from build123d import *

# Parameters (mm, degrees)
ESTRUSIONE_ESTRUSIONE1_DEPTH = 5
ESTRUSIONE_ESTRUSIONE2_DEPTH = 7
ESTRUSIONE_ESTRUSIONE3_DEPTH = 2
ESTRUSIONE_ESTRUSIONE4_DEPTH = 52
TAGLIO_ESTRUSIONE2_DEPTH     = 52
ESTRUSIONE_ESTRUSIONE5_DEPTH = 9
FORI_FILETTATI_3_0MM1_D      = 3


with BuildPart() as part:
    # Schizzo1 → Estrusione-Estrusione1 (new body)
    with BuildSketch(Plane.XY):
        with BuildLine():
            Line((-82.995904107, -166.584374689), (-92.877799089, -168.116742646))
            ThreePointArc((-92.877799089, -168.116742646), (-110.220012955, -164.040092202), (-119.840608042, -149.046239769))
            ThreePointArc((-119.840608042, -149.046239769), (-118.364815633, -130.917411526), (-107.867932944, -116.063192243))
            Line((-107.867932944, -116.063192243), (-84.49215827, -97.259651129))
            ThreePointArc((-84.49215827, -97.259651129), (-67.733683115, -90.189581316), (-49.709718148, -92.632748029))
            ThreePointArc((-49.709718148, -92.632748029), (-37.125664022, -105.242785395), (-36.859828578, -123.055724291))
            Line((-36.859828578, -123.055724291), (-40.474113425, -132.379722631))
            Line((-40.474113425, -132.379722631), (-54.467826156, -126.955304689))
            Line((-54.467826156, -126.955304689), (-50.853541308, -117.631306349))
            ThreePointArc((-50.853541308, -117.631306349), (-51.095893898, -108.22813541), (-57.953355129, -101.789689638))
            ThreePointArc((-57.953355129, -101.789689638), (-68.520842721, -100.735914417), (-78.224311232, -105.051576021))
            Line((-78.224311232, -105.051576021), (-101.600085906, -123.855117134))
            ThreePointArc((-101.600085906, -123.855117134), (-107.894780127, -132.408424149), (-109.129903142, -142.956253658))
            ThreePointArc((-109.129903142, -142.956253658), (-104.310440062, -151.034071069), (-95.177618995, -153.285723315))
            Line((-95.177618995, -153.285723315), (-85.295724012, -151.753355358))
            Line((-85.295724012, -151.753355358), (-82.995904107, -166.584374689))
        make_face()
    extrude(amount=ESTRUSIONE_ESTRUSIONE1_DEPTH)

    # Schizzo2 → Estrusione-Estrusione2 (add)
    with BuildSketch(Plane.XY.offset(5)):
        with BuildLine():
            Line((-36.859828578, -123.055724291), (-50.830842779, -117.640105037))
            ThreePointArc((-50.830842779, -117.640105037), (-50.298673229, -115.886666013), (-50.034997321, -114.073318872))
            Line((-50.034997321, -114.073318872), (-35.811832194, -119.586680021))
            ThreePointArc((-35.811832194, -119.586680021), (-36.269524014, -121.341233275), (-36.859828578, -123.055724291))
        make_face()
        with BuildLine():
            Line((-96.490830562, -168.397042736), (-98.828360202, -153.322841843))
            ThreePointArc((-98.828360202, -153.322841843), (-97.000632762, -153.453858051), (-95.173888567, -153.309779998))
            Line((-95.173888567, -153.309779998), (-92.877799089, -168.116742646))
            ThreePointArc((-92.877799089, -168.116742646), (-94.678957246, -168.325951195), (-96.490830562, -168.397042736))
        make_face()
    extrude(amount=ESTRUSIONE_ESTRUSIONE2_DEPTH)

    # Schizzo3 → Estrusione-Estrusione3 (add)
    with BuildSketch(Plane.XY.offset(12)):
        with BuildLine():
            Line((-42.270578454, -137.014176653), (-36.859828578, -123.055724291))
            ThreePointArc((-36.859828578, -123.055724291), (-36.269524014, -121.341233275), (-35.811832194, -119.586680021))
            Line((-35.811832194, -119.586680021), (-50.034997321, -114.073318872))
            ThreePointArc((-50.034997321, -114.073318872), (-50.288758238, -115.888878313), (-50.830842779, -117.640105037))
            Line((-50.830842779, -117.640105037), (-53.115040991, -123.532795079))
            Line((-53.115040991, -123.532795079), (-42.270578454, -137.014176653))
        make_face()
        with BuildLine():
            Line((-96.490830562, -168.397042736), (-98.828360202, -153.322841843))
            ThreePointArc((-98.828360202, -153.322841843), (-97.000596453, -153.464016791), (-95.173888567, -153.309779998))
            Line((-95.173888567, -153.309779998), (-88.928612449, -152.34133609))
            Line((-88.928612449, -152.34133609), (-78.084149913, -165.822717664))
            Line((-78.084149913, -165.822717664), (-92.877799089, -168.116742646))
            ThreePointArc((-92.877799089, -168.116742646), (-94.678957246, -168.325951195), (-96.490830562, -168.397042736))
        make_face()
    extrude(amount=ESTRUSIONE_ESTRUSIONE3_DEPTH)

    # Schizzo4 → Estrusione-Estrusione4 (add)
    with BuildSketch(Plane.XY.offset(5)):
        Polygon((-101.600085906, -123.855117134), (-78.224311232, -105.051576021), (-84.49215827, -97.259651129), (-107.867932944, -116.063192243), align=None)
    extrude(amount=ESTRUSIONE_ESTRUSIONE4_DEPTH)

    # Schizzo5 → Taglio-Estrusione2 (cut)
    with BuildSketch(Plane.XY.offset(57)):
        Polygon((-97.246900104, -116.503262037), (-97.873684808, -115.724069548), (-98.141552252, -109.009291291), (-98.517623074, -108.541775798), (-93.842468139, -104.781067575), (-93.466397317, -105.248583068), (-86.96498996, -106.949083694), (-86.338205256, -107.728276184), align=None)
    extrude(amount=-TAGLIO_ESTRUSIONE2_DEPTH, mode=Mode.SUBTRACT)

    # Schizzo6 → Estrusione-Estrusione5 (add)
    with BuildSketch(Plane.XY.offset(5)):
        with BuildLine():
            Line((-105.360794128, -119.1799622), (-104.107224721, -120.738347178))
            ThreePointArc((-104.107224721, -120.738347178), (-113.327097811, -135.89060806), (-110.731703589, -153.436576214))
            ThreePointArc((-110.731703589, -153.436576214), (-105.298812913, -158.702833766), (-97.823256998, -159.87152255))
            Line((-97.823256998, -159.87152255), (-97.519846298, -161.848374074))
            ThreePointArc((-97.519846298, -161.848374074), (-106.191101066, -160.49275607), (-112.492970749, -154.384172115))
            ThreePointArc((-112.492970749, -154.384172115), (-115.28727508, -135.493487076), (-105.360794128, -119.1799622))
        make_face()
        with BuildLine():
            Line((-43.853805634, -116.458338954), (-41.987888093, -117.178305432))
            ThreePointArc((-41.987888093, -117.178305432), (-41.453924934, -108.417983362), (-46.070241465, -100.953535552))
            ThreePointArc((-46.070241465, -100.953535552), (-63.923362402, -94.176206375), (-81.985019455, -100.376421086))
            Line((-81.985019455, -100.376421086), (-80.731450047, -101.934806064))
            ThreePointArc((-80.731450047, -101.934806064), (-63.955496248, -96.175948212), (-47.373234104, -102.470839142))
            ThreePointArc((-47.373234104, -102.470839142), (-43.393471858, -108.905997429), (-43.853805634, -116.458338954))
        make_face()
    extrude(amount=ESTRUSIONE_ESTRUSIONE5_DEPTH)

    # Fori filettati Ø3.0mm1 (through all)
    with Locations(Plane.XY.offset(14)):
        with Locations((-88.877799089, -160.412808131), (-44.832341355, -124.255324234)):
            Hole(FORI_FILETTATI_3_0MM1_D / 2)


solid = part.part
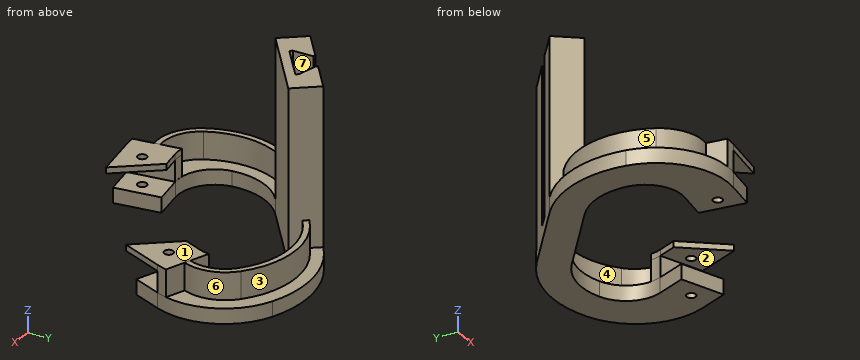
Work out the finished part from the listing and answer in its coordinate system (mm). Face numbers are marked on the shaded views. A direction names the side the tool comes from. Round coordinates to 2 decimals unless told otherwise and drop trailing zeros. Write each loop counter-clockwise with the first axis right and the second up, starting at its lowest first coordinate (ties: lowest second). Pieces come first, ordered by that corner, then holes.
1) Straight lines are drawn through the part: line 1 (X direction, y = -99, z = 13); line 2 (Z direction, x = -46, y = -122); line 3 (Z direction, x = -51.5, y = -98). For each, find the intervals that lie inside material, in ascending order.
2) The mould has two halves that part along X. Classify the marked faces 5, 6 and 7: pulls with the +X half, pulls with the -X half, needs draft (parallel to the pull), parting line crosses it, or undercut.
3) A cutting plane is placed at C-C (z = 9). Give the number of separate pieces and of enclosed holes in the cut face, plus the area to 3 significant figures.
4) A cutting plane is placed at B-B (x = -103). Give the vertices of the cut face in (y, z).
5) A cutting plane is placed at D-D (x = -64). Give the vertices of the cut face in (y, z), plus the area to 3 significant figures.
6) Given pin 1 Ø1 at (x, y) = (-74.5, -99) entering from +Z; pin 2 Ø5 at (y, z) = (-98.5, 29.5) entering from +X; pin 3 Ø3.5 at (x, y) = (-44.83, -124.26) entering from +Z; pin 4 Ø5 at (x, y) = (-41.5, -132) entering from -Z, each flat-ended and moving along its own axis, determine where each tip first touches the part or whether it passes through.
7) A tool of negligible diameter and unlimited length cuts with its end or side. For the marked faces 1, 2, 3 and 4, from which of +Z, -Z, +X, -X, +Y, -Y can it reach the whole face along a straight path? Write none if from no direction.
8) A cutting plane is placed at A-A (z = 24.5). Give the vertices of the cut face in (x, y).
Completed:
1. line 1: x = -86.66 to -83.09, -80.12 to -76.19, -52.56 to -48.63
1. line 2: z = 0 to 5, 12 to 14
1. line 3: z = 0 to 14
2. face 5: pulls with the -X half
2. face 6: pulls with the +X half
2. face 7: undercut
3. separate pieces: 3
3. enclosed holes: 0
3. area: 554 mm2
4. outline: (-167.49, 0) - (-151.88, 0) - (-151.88, 5) - (-159.58, 5) - (-159.58, 14) - (-161.64, 14) - (-161.64, 5) - (-167.49, 5) - close; (-125.09, 0) - (-112.15, 0) - (-112.15, 57) - (-122.11, 57) - (-122.11, 5) - (-125.09, 5) - close
5. outline: (-100.51, 0) - (-89.9, 0) - (-89.9, 5) - (-94.18, 5) - (-94.18, 14) - (-96.18, 14) - (-96.18, 5) - (-100.51, 5) - close
5. area: 71.1 mm2
6. pin 1: stops at z = 5
6. pin 2: stops at x = -81.48
6. pin 3: stops at z = 14
6. pin 4: stops at z = 0
7. face 1: +Z, +X, +Y, -Y
7. face 2: -Y
7. face 3: +Z, +Y
7. face 4: +Z
8. outline: (-107.87, -116.06) - (-101.6, -123.86) - (-78.22, -105.05) - (-84.49, -97.26) - (-93.84, -104.78) - (-93.47, -105.25) - (-86.96, -106.95) - (-86.34, -107.73) - (-97.25, -116.5) - (-97.87, -115.72) - (-98.14, -109.01) - (-98.52, -108.54) - close
